from build123d import *

# Parameters (mm, degrees)
PAD010_DEPTH    = 3
SKETCH023_R     = 1.7
HOLE002_DEPTH   = 3
HOLE002_TIPS_R  = 1.7
SKETCH024_R     = 3
POCKET007_DEPTH = 1.5
CHAMFER001_SIZE = 1


with BuildPart() as part:
    # Sketch022 (on Face1 of CopyPad011) → Pad010 (new body)
    with BuildSketch(Plane.XY.offset(24)):
        Polygon((-3, -6), (70, -6), (78, -16), (108, -16), (108, 70), (-3, 70), align=None)
    extrude(amount=PAD010_DEPTH)

    # Sketch023 (on Face8 of Pad010) → Hole002 (cut)
    with BuildSketch(Plane.XY.offset(27)):
        with Locations((1.5, 65.5)):
            Circle(SKETCH023_R)
        with Locations((87.5, 65.5)):
            Circle(SKETCH023_R)
        with Locations((87.5, -11.5)):
            Circle(SKETCH023_R)
        with Locations((1.5, -1.5)):
            Circle(SKETCH023_R)
    extrude(amount=-HOLE002_DEPTH, mode=Mode.SUBTRACT)

    # Hole002 tips → Hole002 tip 1 section 0
    with BuildSketch(Plane.XY.offset(24), mode=Mode.PRIVATE) as hole002_tip_1_s0:
        with Locations((1.5, 65.5)):
            Circle(HOLE002_TIPS_R)
    loft([hole002_tip_1_s0.sketch, Vertex(1.5, 65.5, 22.978537)], mode=Mode.SUBTRACT)

    # Hole002 tips → Hole002 tip 2 section 0
    with BuildSketch(Plane.XY.offset(24), mode=Mode.PRIVATE) as hole002_tip_2_s0:
        with Locations((87.5, 65.5)):
            Circle(HOLE002_TIPS_R)
    loft([hole002_tip_2_s0.sketch, Vertex(87.5, 65.5, 22.978537)], mode=Mode.SUBTRACT)

    # Hole002 tips → Hole002 tip 3 section 0
    with BuildSketch(Plane.XY.offset(24), mode=Mode.PRIVATE) as hole002_tip_3_s0:
        with Locations((87.5, -11.5)):
            Circle(HOLE002_TIPS_R)
    loft([hole002_tip_3_s0.sketch, Vertex(87.5, -11.5, 22.978537)], mode=Mode.SUBTRACT)

    # Hole002 tips → Hole002 tip 4 section 0
    with BuildSketch(Plane.XY.offset(24), mode=Mode.PRIVATE) as hole002_tip_4_s0:
        with Locations((1.5, -1.5)):
            Circle(HOLE002_TIPS_R)
    loft([hole002_tip_4_s0.sketch, Vertex(1.5, -1.5, 22.978537)], mode=Mode.SUBTRACT)

    # Sketch024 (on Face5 of Hole002) → Pocket007 (cut)
    with BuildSketch(Plane.XY.offset(27)):
        with Locations((1.5, 65.5)):
            Circle(SKETCH024_R)
        with Locations((87.5, 65.5)):
            Circle(SKETCH024_R)
        with Locations((87.5, -11.5)):
            Circle(SKETCH024_R)
        with Locations((1.5, -1.5)):
            Circle(SKETCH024_R)
    extrude(amount=-POCKET007_DEPTH, mode=Mode.SUBTRACT)

    # Chamfer001
    chamfer001_edges = [part.edges().sort_by_distance(p)[0] for p in [
        (-3, -6, 25.5),
        (-3, 32, 27),
        (33.5, -6, 27),
        (93, -16, 27),
        (74, -11, 27),
        (108, 27, 27),
        (52.5, 70, 27),
        (108, -16, 25.5),
        (108, 70, 25.5),
        (-3, 70, 25.5),
    ]]
    chamfer(chamfer001_edges, length=CHAMFER001_SIZE)


with BuildPart() as part_1:
    # Body002 placement: moved
    add(part.part.moved(Location((0, 0, -2.5))))


solid = part_1.part
Verification items for the finished model (mm, model axes). A direction names the side the tool comes from. Coordinates: 2 decimals unless noted, no trailing zeros. Order: outer loops, then holes, each group sorted by start corner. A loop starts at its lowest first (then second) coordinate and runs counter-clockwise, first axis right, second up.
1. Sectioned sample at B-B, the plane y = 65.5. Record the cut outline in (x, z).
Results found:
outline: (-3, 21.5) - (-0.2, 21.5) - (-0.2, 23) - (-1.5, 23) - (-1.5, 24.5) - (-2, 24.5) - (-3, 23.5) - close; (3.2, 21.5) - (85.8, 21.5) - (85.8, 23) - (84.5, 23) - (84.5, 24.5) - (4.5, 24.5) - (4.5, 23) - (3.2, 23) - close; (89.2, 21.5) - (108, 21.5) - (108, 23.5) - (107, 24.5) - (90.5, 24.5) - (90.5, 23) - (89.2, 23) - close
2. Go/stop test with flat-tipped pins: pin 1 Ø3 at (x, y) = (1.5, -2) entering from +Z; pin 2 Ø0.6 at (x, z) = (47.5, 22.5) entering from -Y. Record where each tip stops, or that it passes through.
Results found:
pin 1: stops at z = 23
pin 2: stops at y = -6
3. Set-up check for faces 5 (the face through (84.5, -11.4, 23.8)), 6 (the face through (74, -11, 22)): record each of +Z, -Z, +X, -X, +Y, -Y from which the full face is reachable in a straight line by a thin tool's end or side.
Results found:
face 5: +Z
face 6: +Z, -Z, -X, -Y
4. Sectioned sample at A-A, the plane x = 87.5. Record the cut outline in (y, z), and give its area (3 significant figures).
Results found:
outline: (-16, 21.5) - (-13.2, 21.5) - (-13.2, 23) - (-14.5, 23) - (-14.5, 24.5) - (-15, 24.5) - (-16, 23.5) - close; (-9.8, 21.5) - (63.8, 21.5) - (63.8, 23) - (62.5, 23) - (62.5, 24.5) - (-8.5, 24.5) - (-8.5, 23) - (-9.8, 23) - close; (67.2, 21.5) - (70, 21.5) - (70, 23.5) - (69, 24.5) - (68.5, 24.5) - (68.5, 23) - (67.2, 23) - close
area: 229 mm2
5. Release check for a two-part mould opening along X. For faces 1 (the face through (52, 28, 21.5)), 2 (the face through (74.19, -10.42, 24.01)), 3 (the face through (3, 64, 23)), 4 (the face through (3.12, -0.99, 22.26)) record: +X half, -X half, draft (parallel to the pull), parting line (faces both ways), or undercut.
Results found:
face 1: draft
face 2: -X half
face 3: undercut
face 4: undercut
6. Scan lines: line 1 (Y direction, x = 87.5, z = 22); line 2 (Y direction, x = 1.5, z = 22); line 3 (Y direction, x = 46, z = 22.3). Record each from-to range of solid material in increasing order.
Results found:
line 1: y = -16 to -13.2, -9.8 to 63.8, 67.2 to 70
line 2: y = -6 to -3.2, 0.2 to 63.8, 67.2 to 70
line 3: y = -6 to 70
7. Sectioned sample at D-D, the plane z = 22.5. Record the cut outline in (x, y), and give its area (3 significant figures).
Results found:
outline: (-3, -5) - (-2, -6) - (70, -6) - (78, -16) - (107, -16) - (108, -15) - (108, 69) - (107, 70) - (-2, 70) - (-3, 69) - close; hole circle Ø3.4 at (1.5, -1.5); hole circle Ø3.4 at (1.5, 65.5); hole circle Ø3.4 at (87.5, -11.5); hole circle Ø3.4 at (87.5, 65.5)
area: 8,740 mm2
8. Sectioned sample at C-C, the plane y = -11.5. Record the cut outline in (x, z), and give its area (3 significant figures).
Results found:
outline: (74.4, 21.5) - (85.8, 21.5) - (85.8, 23) - (84.5, 23) - (84.5, 24.5) - (75.68, 24.5) - (74.4, 23.5) - close; (89.2, 21.5) - (108, 21.5) - (108, 23.5) - (107, 24.5) - (90.5, 24.5) - (90.5, 23) - (89.2, 23) - close
area: 85.6 mm2
